Input: part model. Units: mm. Frame: model coordinates. A direction names the side the tool comes from. Coordinates: 2 decimals unless noted, no trailing zeros. Loops run counter-clockwise (first coordinate to the right, second up) from the corner with the lowest first, then second, coordinate; pieces in that order, holes last. Notation, with made-up numbers: M -27,48 L 21,48 A18 ccw 21,83 Z; hole C 62,68 d11. An arc over 180 degrees is marked long. Use a Markdown table: item, result. Add a question column.
1. Section D-D on y = -0.75. Output: boundary loops of the cut face in (x, z), then the cut area to 3 significant figures.
2. Section A-A on z = 3.25. State how many separate pieces and enclosed holes the cut face has, then the cut area to 3 significant figures.
3. Set-up query: faces 1 (the flat face through (7, -5, -2)), 2 (the flat face through (12, -5, 6)), 3 (the flat face through (9.6, -2.7, 6)), 4 (the cylindrical face through (9.173, -5.078, -1.014)). Return all of +Z, -Z, +X, -X, +Y, -Y with unobstructed straight access to the full face (end or side cutting, diameter ignored); none if empty.
4. Pin query (flat end, axial travel): pin 1 (0.8 mm diameter, centred on x = 9.5, y = -5, fed in from +Z); pin 2 (2 mm diameter, centred on y = -2, z = 2.5, fed in from -X). Return the tip coordinate at first contact, or that it passes through.
5. Section B-B on z = 6.25. Output: boundary loops of the cut face in (x, y) (3 decimals).
6. Section C-C on x = 13.5. Output: boundary loops of the cut face in (y, z).
7. Draft query along X for faces 5 (the cylindrical face through (4.952, -2.426, -1.014)), 6 (the flat face through (10, 0, 3)). Return one class per face: +X half, -X half, draft (parallel to the pull), parting line (faces both ways), or undercut.
8. Line query: L1, parallel to Y at x = 17.5, z = 4.5; L2, parallel to X at y = -6.25, z = 2; L3, parallel to Y at x = 9.75, z = 2.25. Output: solid intervals per line, ascending. Write a range as [from, to].
```python
from build123d import *

# Parameters (mm, degrees)
SKETCH_1_W           = 19.27
SKETCH_1_H           = 8
EXTRUDE_1_DEPTH      = 7
SKETCH_2_W           = 17.27
SKETCH_2_H           = 6
CUT_EXTRUDE_1_DEPTH  = 6
CUT_EXTRUDE_2_REACH  = 24.008
EXTRUDE_2_DEPTH      = 5
EXTRUDE_2_DEPTH_BACK = 3
SKETCH_4_R           = 0.5


with BuildPart() as part:
    # 草图1 → 凸台-拉伸1 (new body)
    with BuildSketch(Plane.XY):
        with Locations((9.635, -4)):
            Rectangle(SKETCH_1_W, SKETCH_1_H)
    extrude(amount=EXTRUDE_1_DEPTH)

    # 草图2 → 切除-拉伸1 (cut)
    with BuildSketch(Plane.XY.offset(7)):
        with Locations((9.635, -4)):
            Rectangle(SKETCH_2_W, SKETCH_2_H)
    extrude(amount=-CUT_EXTRUDE_1_DEPTH, mode=Mode.SUBTRACT)

    # 草图3 → 切除-拉伸2 (cut, up to next)
    with BuildSketch(Plane.XZ.offset(8), mode=Mode.PRIVATE) as cut_extrude_2_sk1:
        Polygon((8.365, 7), (8.365, 4.46), (9.635, 4), (10.905, 4.46), (10.905, 7), align=None)
    cut_extrude_2_tool1 = extrude(cut_extrude_2_sk1.sketch, amount=-CUT_EXTRUDE_2_REACH, mode=Mode.PRIVATE) & part.part
    add(cut_extrude_2_tool1.solids().sort_by_distance((9.635, -8, 5.611817))[0], mode=Mode.SUBTRACT)

    # 草图4 → 凸台-拉伸2 (add, two sides: drawn at the far end of the back side and taken through both)
    with BuildSketch(Plane.XY.offset(1).offset(-EXTRUDE_2_DEPTH_BACK)):
        with Locations((9.635, -2.73)):
            Circle(SKETCH_4_R)
        with Locations((12.175, -2.73)):
            Circle(SKETCH_4_R)
        with Locations((14.715, -2.73)):
            Circle(SKETCH_4_R)
        with Locations(Location((4.555, -2.73, 0), (0, 0, 180))):
            Circle(SKETCH_4_R)
        with Locations(Location((7.095, -2.73, 0), (0, 0, 180))):
            Circle(SKETCH_4_R)
        with Locations(Location((14.715, -5.27, 0), (0, 0, 180))):
            Circle(SKETCH_4_R)
        with Locations(Location((12.175, -5.27, 0), (0, 0, 180))):
            Circle(SKETCH_4_R)
        with Locations(Location((9.635, -5.27, 0), (0, 0, 180))):
            Circle(SKETCH_4_R)
        with Locations((7.095, -5.27)):
            Circle(SKETCH_4_R)
        with Locations((4.555, -5.27)):
            Circle(SKETCH_4_R)
    extrude(amount=EXTRUDE_2_DEPTH + EXTRUDE_2_DEPTH_BACK)


solid = part.part
```
Answers below:
| question | item | result |
|---|---|---|
| 1 | outline | M 0,0 L 19.27,0 L 19.27,7 L 0,7 Z |
| 1 | area | 135 mm² |
| 2 | separate pieces | 11 |
| 2 | enclosed holes | 1 |
| 2 | area | 58.4 mm² |
| 3 | face 1 | -Z, +X, -X, +Y, -Y |
| 3 | face 2 | +Z |
| 3 | face 3 | +Z, -Y |
| 3 | face 4 | -Z |
| 4 | pin 1 | stops at z = 6 |
| 4 | pin 2 | stops at x = 0 |
| 5 | outline | M 0,-8 L 8.365,-8 L 8.365,-7 L 1,-7 L 1,-1 L 18.27,-1 L 18.27,-7 L 10.905,-7 L 10.905,-8 L 19.27,-8 L 19.27,0 L 0,0 Z |
| 6 | outline | M -8,0 L 0,0 L 0,7 L -1,7 L -1,1 L -7,1 L -7,7 L -8,7 Z |
| 7 | face 5 | undercut |
| 7 | face 6 | draft |
| 8 | L1 | y = [-8, -7], [-1, 0] |
| 8 | L2 | x = [0, 1], [18.27, 19.27] |
| 8 | L3 | y = [-8, -7], [-5.76, -4.78], [-3.22, -2.24], [-1, 0] |
